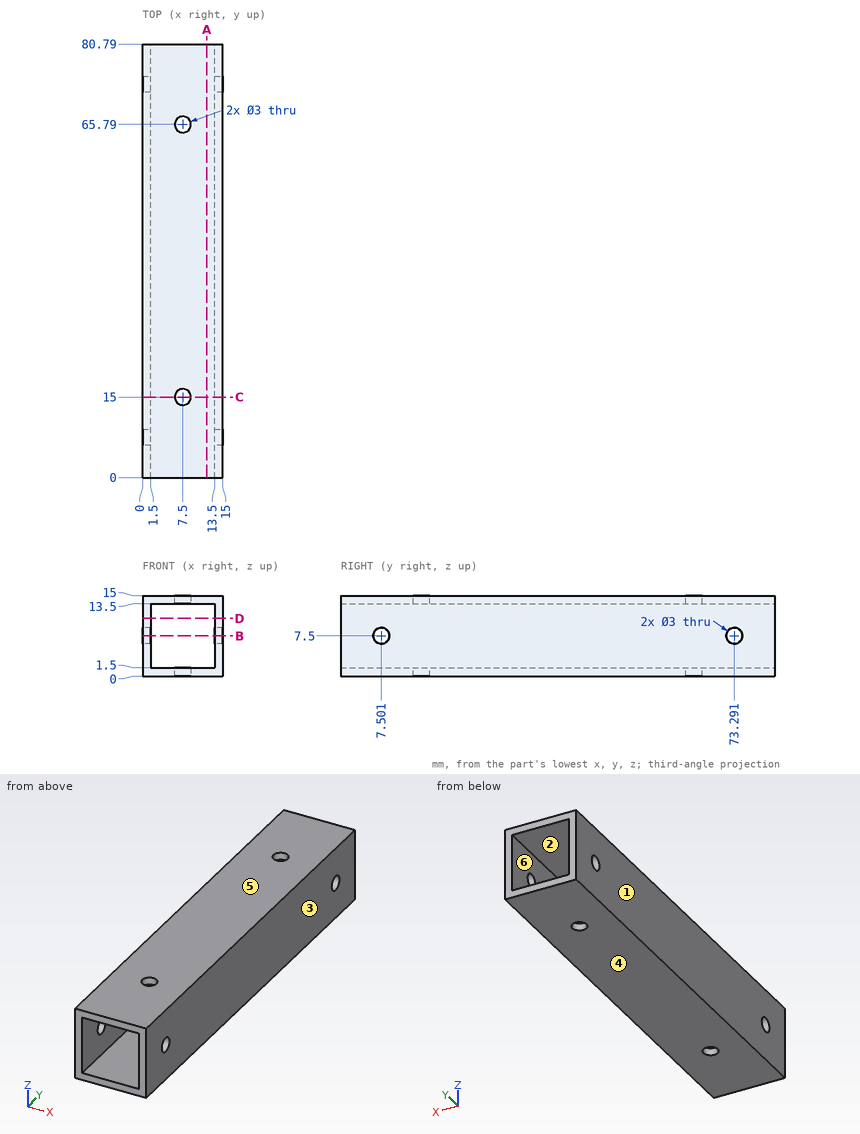
Source: three-view drawing plus pictorial views. Frame: mm from the lowest corner of the part. A direction names the side the tool comes from. Coordinates: 2 decimals unless noted, no trailing zeros. Order: outer loops, then holes, each group sorted by start corner. A loop starts at its lowest first (then second) coordinate and runs counter-clockwise, first axis right, second up. Notation, with made-up numbers: M 81,37 L 88,37 A20 cw 88,71 Z; hole C 61.25,37 d8. An arc over 180 degrees is marked long. Write each question's results on one line, items separated by ' | '. Start each with the question number.
1. Reachability of the marked faces 5 and 6 from +Z, -Z, +X, -X, +Y, -Y: full face, straight path, thin tool, end or side. Return the list, or none.
2. Section C-C, the plane y = 15. Return the cut outline in (x, z).
3. Section A-A, the plane x = 12. Return the cut outline in (y, z).
4. Pin query (flat end, axial travel): pin 1 (5 mm diameter, centred on y = 19, z = 10, fed in from -X); pin 2 (2.5 mm diameter, centred on x = 7.5, y = 15, fed in from +Z). Return the tip coordinate at first contact, or that it passes through.
5. Material intervals for L1, parallel to Y at x = 7.5, z = 14.4; L2, parallel to Z at x = 6.5, y = 52, sorted ascending.
6. Draft query along X for the marked faces 1, 2, 3 and 4. Return one class per face: +X half, -X half, draft (parallel to the pull), parting line (faces both ways), or undercut.
7. Section D-D, the plane z = 10.75. Return the cut outline in (x, y).
8. Section B-B, the plane z = 7.5. Return the cut outline in (x, y).
Solution:
1) face 5: +Z, +X, -X, +Y, -Y | face 6: +Y, -Y
2) outline: M 0,0 L 6,0 L 6,1.5 L 1.5,1.5 L 1.5,13.5 L 6,13.5 L 6,15 L 0,15 Z; M 9,0 L 15,0 L 15,15 L 9,15 L 9,13.5 L 13.5,13.5 L 13.5,1.5 L 9,1.5 Z
3) outline: M 0,0 L 80.79,0 L 80.79,1.5 L 0,1.5 Z; M 0,13.5 L 80.79,13.5 L 80.79,15 L 0,15 Z
4) pin 1: x = 0 | pin 2: through
5) L1: 0 to 13.5, 16.5 to 64.29, 67.29 to 80.79 | L2: 0 to 1.5, 13.5 to 15
6) face 1: -X half | face 2: undercut | face 3: +X half | face 4: draft
7) outline: M 0,0 L 1.5,0 L 1.5,80.79 L 0,80.79 Z; M 13.5,0 L 15,0 L 15,80.79 L 13.5,80.79 Z
8) outline: M 0,0 L 1.5,0 L 1.5,6 L 0,6 Z; M 0,9 L 1.5,9 L 1.5,71.79 L 0,71.79 Z; M 0,74.79 L 1.5,74.79 L 1.5,80.79 L 0,80.79 Z; M 13.5,0 L 15,0 L 15,6 L 13.5,6 Z; M 13.5,9 L 15,9 L 15,71.79 L 13.5,71.79 Z; M 13.5,74.79 L 15,74.79 L 15,80.79 L 13.5,80.79 Z
